Geometry check sheet. Reference: the model listing, model coordinates, mm. A direction names the side the tool comes from. Round coordinates to 2 decimals unless told otherwise and drop trailing zeros. Order: outer loops, then holes, each group sorted by start corner. A loop starts at its lowest first (then second) coordinate and runs counter-clockwise, first axis right, second up.
(1) Sectioned sample at D-D (y = -2.75). Record the boundary of the cut face in (x, z).
(2) Sectioned sample at A-A (y = 0). Record the boundary of the cut face in (x, z).
(3) Set-up check for faces 1 (the face through (14.23, -0.91, 2.94)), 2 (the face through (0, 10, 2)): record each of +Z, -Z, +X, -X, +Y, -Y from which the full face is reachable in a straight line by a thin tool's end or side.
(4) Go/stop test with a flat-tipped pin: pin 1 (2 mm diameter, centred on y = 4.5, z = 2, fed in from +X). Record where the tip stops, or that it passes through.
(5) Sectioned sample at B-B (z = 1.75). Record the boundary of the cut face in (x, y), plus the area to 3 significant figures.
(6) Sectioned sample at C-C (x = -2.5). Record the boundary of the cut face in (y, z), plus the area to 4 significant figures.
(7) Material ranges on line 1 along Y through (x, z) = (-2.5, 1.3); line 2 along X through (y, z) = (5.75, 1.25); line 3 along X through (y, z) = (-1, 1.5), recorded low to high.
from build123d import *

# Parameters (mm, degrees)
SKETCH_1_W      = 25
SKETCH_1_H      = 20
SKETCH_1_R      = 1.55
EXTRUDE_1_DEPTH = 3.5
SKETCH_2_R      = 1.5
EXTRUDE_2_DEPTH = 3.5


with BuildPart() as part:
    # 草图1 → 凸台-拉伸1 (new body)
    with BuildSketch(Plane.XY):
        Rectangle(SKETCH_1_W, SKETCH_1_H)
        with Locations((-2.5, 0)):
            Circle(SKETCH_1_R, mode=Mode.SUBTRACT)
    extrude(amount=EXTRUDE_1_DEPTH)

    # 草图2 → 凸台-拉伸2 (add)
    with BuildSketch(Plane(origin=(12.5, 0, 0), x_dir=(0, 0, -1), z_dir=(1, 0, 0))):
        with Locations((-1.75, 0)):
            Circle(SKETCH_2_R)
    extrude(amount=EXTRUDE_2_DEPTH)


solid = part.part
Answer below:
1. outline: (-12.5, 0) - (12.5, 0) - (12.5, 3.5) - (-12.5, 3.5) - close
2. outline: (-12.5, 0) - (-4.05, 0) - (-4.05, 3.5) - (-12.5, 3.5) - close; (-0.95, 0) - (12.5, 0) - (12.5, 0.25) - (16, 0.25) - (16, 3.25) - (12.5, 3.25) - (12.5, 3.5) - (-0.95, 3.5) - close
3. face 1: +X
3. face 2: +Z, -Z, +X, -X, +Y
4. pin 1: stops at x = 12.5
5. outline: (-12.5, -10) - (12.5, -10) - (12.5, -1.5) - (16, -1.5) - (16, 1.5) - (12.5, 1.5) - (12.5, 10) - (-12.5, 10) - close; hole circle Ø3.1 at (-2.5, 0)
5. area: 503 mm2
6. outline: (-10, 0) - (-1.55, 0) - (-1.55, 3.5) - (-10, 3.5) - close; (1.55, 0) - (10, 0) - (10, 3.5) - (1.55, 3.5) - close
6. area: 59.15 mm2
7. line 1: y = -10 to -1.55, 1.55 to 10
7. line 2: x = -12.5 to 12.5
7. line 3: x = -12.5 to -3.68, -1.32 to 16
